Geometry: final body of the model. Coordinates: model frame, mm. Round coordinates to 2 decimals unless told otherwise and drop trailing zeros. Loops run counter-clockwise (first coordinate to the right, second up) from the corner with the lowest first, then second, coordinate; pieces in that order, holes last. Notation, with made-up numbers: M 14,-14 L 64,-14 A10 ccw 64,2 Z; hole C 22.25,43 d4. An arc over 180 degrees is marked long. Answer as a JSON object with one key per item and string values.
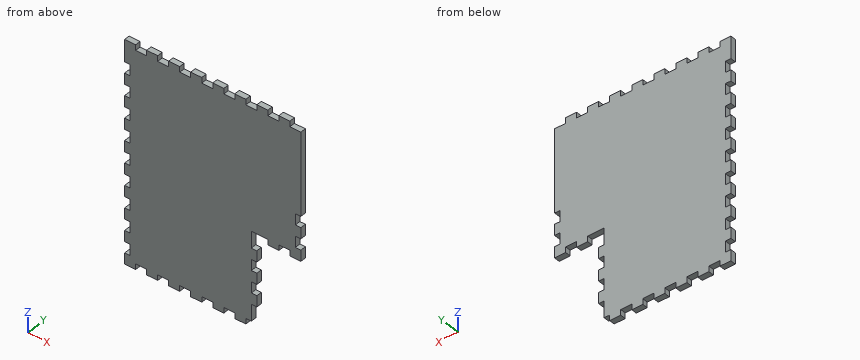
from build123d import *

# Parameters (mm, degrees)
SKETCH1_W           = 203.2
SKETCH1_H           = 254
BOSS_EXTRUDE1_DEPTH = 6.35
SKETCH2_W           = 50.8
SKETCH2_H           = 101.6
CUT_EXTRUDE2_DEPTH  = 7.35
SKETCH3_W           = 12.7
SKETCH3_H           = 6.35
CUT_EXTRUDE3_DEPTH  = 7.35
LPATTERN1_COUNT     = 8
LPATTERN1_PITCH     = 25.4
SKETCH4_W           = 6.35
SKETCH4_H           = 12.7
CUT_EXTRUDE4_DEPTH  = 7.35
LPATTERN2_COUNT     = 9
LPATTERN2_PITCH     = 25.4
SKETCH5_W           = 12.7
SKETCH5_H           = 6.35
CUT_EXTRUDE5_DEPTH  = 7.35
LPATTERN3_COUNT     = 6
LPATTERN3_PITCH     = 25.4
SKETCH7_W           = 6.35
SKETCH7_H           = 12.7
CUT_EXTRUDE8_DEPTH  = 7.35
LPATTERN5_COUNT     = 2
LPATTERN5_PITCH     = 25.4
SKETCH8_W           = 12.7
SKETCH8_H           = 6.35
CUT_EXTRUDE9_DEPTH  = 7.35
LPATTERN6_COUNT     = 2
LPATTERN6_PITCH     = 25.4
SKETCH9_W           = 6.35
SKETCH9_H           = 19.05
CUT_EXTRUDE10_DEPTH = 7.35
SKETCH10_W          = 6.35
SKETCH10_H          = 12.7
CUT_EXTRUDE11_DEPTH = 7.35
LPATTERN7_COUNT     = 3
LPATTERN7_PITCH     = 25.4
SKETCH11_W          = 6.35
SKETCH11_H          = 6.35
CUT_EXTRUDE12_DEPTH = 7.35


with BuildPart() as part:
    # Sketch1 → Boss-Extrude1 (new body)
    with BuildSketch(Plane(origin=(0, 0, 0), x_dir=(1, 0, 0), z_dir=(0, 1, 0))):
        Rectangle(SKETCH1_W, SKETCH1_H)
    extrude(amount=BOSS_EXTRUDE1_DEPTH)

    # Sketch2 → Cut-Extrude2 (cut, through all)
    with BuildSketch(Plane(origin=(0, 6.35, 0), x_dir=(1, 0, 0), z_dir=(0, 1, 0))):
        with Locations((76.2, 76.2)):
            Rectangle(SKETCH2_W, SKETCH2_H)
    extrude(amount=-CUT_EXTRUDE2_DEPTH, mode=Mode.SUBTRACT)

    # Sketch3 → Cut-Extrude3 (cut, through all)
    with BuildSketch(Plane(origin=(0, 6.35, 0), x_dir=(1, 0, 0), z_dir=(0, 1, 0))):
        with Locations((95.25, -123.825)):
            Rectangle(SKETCH3_W, SKETCH3_H)
    cut_extrude3 = extrude(amount=-CUT_EXTRUDE3_DEPTH, mode=Mode.SUBTRACT)

    # LPattern1: Cut-Extrude3 ×8
    with Locations(*[(-i * LPATTERN1_PITCH, 0, 0) for i in range(1, LPATTERN1_COUNT)]):
        add(cut_extrude3, mode=Mode.SUBTRACT)

    # Sketch4 → Cut-Extrude4 (cut, through all)
    with BuildSketch(Plane(origin=(0, 6.35, 0), x_dir=(1, 0, 0), z_dir=(0, 1, 0))):
        with Locations((-98.425, -95.25)):
            Rectangle(SKETCH4_W, SKETCH4_H)
    cut_extrude4 = extrude(amount=-CUT_EXTRUDE4_DEPTH, mode=Mode.SUBTRACT)

    # LPattern2: Cut-Extrude4 ×9
    with Locations(*[(0, 0, -i * LPATTERN2_PITCH) for i in range(1, LPATTERN2_COUNT)]):
        add(cut_extrude4, mode=Mode.SUBTRACT)

    # Sketch5 → Cut-Extrude5 (cut, through all)
    with BuildSketch(Plane(origin=(0, 6.35, 0), x_dir=(1, 0, 0), z_dir=(0, 1, 0))):
        with Locations((44.45, 123.825)):
            Rectangle(SKETCH5_W, SKETCH5_H)
    cut_extrude5 = extrude(amount=-CUT_EXTRUDE5_DEPTH, mode=Mode.SUBTRACT)

    # LPattern3: Cut-Extrude5 ×6
    with Locations(*[(-i * LPATTERN3_PITCH, 0, 0) for i in range(1, LPATTERN3_COUNT)]):
        add(cut_extrude5, mode=Mode.SUBTRACT)

    # Sketch7 → Cut-Extrude8 (cut, through all)
    with BuildSketch(Plane(origin=(0, 6.35, 0), x_dir=(1, 0, 0), z_dir=(0, 1, 0))):
        with Locations((98.425, 6.35)):
            Rectangle(SKETCH7_W, SKETCH7_H)
    cut_extrude8 = extrude(amount=-CUT_EXTRUDE8_DEPTH, mode=Mode.SUBTRACT)

    # LPattern5: Cut-Extrude8 ×2
    with Locations(*[(0, 0, i * LPATTERN5_PITCH) for i in range(1, LPATTERN5_COUNT)]):
        add(cut_extrude8, mode=Mode.SUBTRACT)

    # Sketch8 → Cut-Extrude9 (cut, through all)
    with BuildSketch(Plane(origin=(0, 6.35, 0), x_dir=(1, 0, 0), z_dir=(0, 1, 0))):
        with Locations((82.55, 22.225)):
            Rectangle(SKETCH8_W, SKETCH8_H)
    cut_extrude9 = extrude(amount=-CUT_EXTRUDE9_DEPTH, mode=Mode.SUBTRACT)

    # LPattern6: Cut-Extrude9 ×2
    with Locations(*[(-i * LPATTERN6_PITCH, 0, 0) for i in range(1, LPATTERN6_COUNT)]):
        add(cut_extrude9, mode=Mode.SUBTRACT)

    # Sketch9 → Cut-Extrude10 (cut, through all)
    with BuildSketch(Plane(origin=(0, 6.35, 0), x_dir=(1, 0, 0), z_dir=(0, 1, 0))):
        with Locations((47.625, 111.125)):
            Rectangle(SKETCH9_W, SKETCH9_H)
    extrude(amount=-CUT_EXTRUDE10_DEPTH, mode=Mode.SUBTRACT)

    # Sketch10 → Cut-Extrude11 (cut, through all)
    with BuildSketch(Plane(origin=(0, 6.35, 0), x_dir=(1, 0, 0), z_dir=(0, 1, 0))):
        with Locations((47.625, 82.55)):
            Rectangle(SKETCH10_W, SKETCH10_H)
    cut_extrude11 = extrude(amount=-CUT_EXTRUDE11_DEPTH, mode=Mode.SUBTRACT)

    # LPattern7: Cut-Extrude11 ×3
    with Locations(*[(0, 0, i * LPATTERN7_PITCH) for i in range(1, LPATTERN7_COUNT)]):
        add(cut_extrude11, mode=Mode.SUBTRACT)

    # Sketch11 → Cut-Extrude12 (cut, through all)
    with BuildSketch(Plane(origin=(0, 6.35, 0), x_dir=(1, 0, 0), z_dir=(0, 1, 0))):
        with Locations((47.625, 22.225)):
            Rectangle(SKETCH11_W, SKETCH11_H)
    extrude(amount=-CUT_EXTRUDE12_DEPTH, mode=Mode.SUBTRACT)


solid = part.part
1) Ray query, line 1 (Z direction, x = 45.5, y = 2); line 2 (X direction, y = 2.25, z = -111); line 3 (X direction, y = 3, z = 46). Return the intervals inside material, ascending.
Results:
{"line 1": "-101.6 to -88.9, -76.2 to -63.5, -50.8 to -38.1, -19.05 to 120.65", "line 2": "-95.25 to 44.45", "line 3": "-95.25 to 101.6"}
2) Section query A-A (x = 20.5). Return the cut outline in (y, z), and give its area (3 significant figures).
Results:
{"outline": "M 0,-120.65 L 6.35,-120.65 L 6.35,120.65 L 0,120.65 Z", "area": "1,530 mm2"}
3) Section query B-B (z = -29). Return the cut outline in (x, y).
Results:
{"outline": "M -95.25,0 L 44.45,0 L 44.45,6.35 L -95.25,6.35 Z"}
4) Pin query (flat end, axial travel): P1, Ø3, axis at x = 47, y = 4, coming from the +Z side; P2, Ø1.9, axis at y = 4, z = 125, coming from the +X side. Return the tip coordinate at first contact, or that it passes through.
Results:
{"P1": "z = 120.65", "P2": "x = 88.9"}
